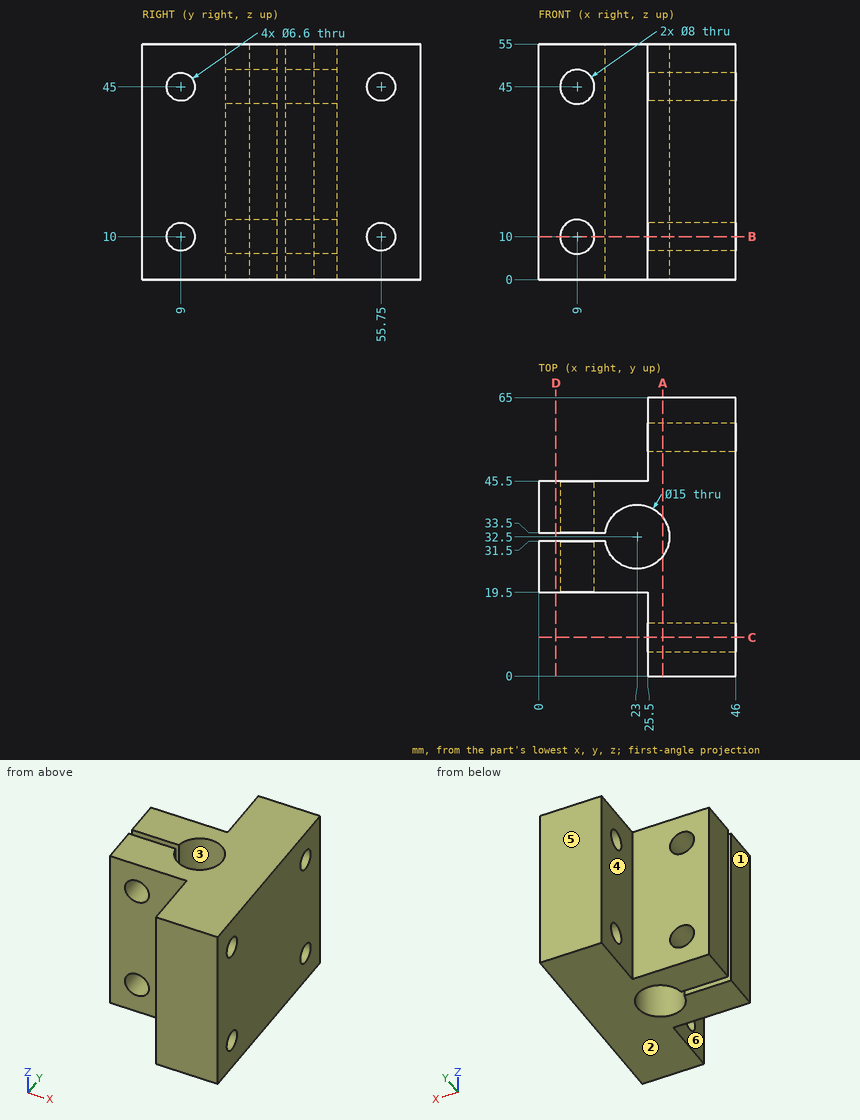
Source: three-view drawing plus pictorial views. Frame: mm from the lowest corner of the part. A direction names the side the tool comes from. Coordinates: 2 decimals unless noted, no trailing zeros. Order: outer loops, then holes, each group sorted by start corner. A loop starts at its lowest first (then second) coordinate and runs counter-clockwise, first axis right, second up. Notation, with made-up numbers: M -24.75,81.25 L -18.75,81.25 A26 ccw -18.75,97.25 Z; hole C 22,19 d3. An arc over 180 degrees is marked long. Write each question's results on one line, items separated by ' | '. Start each with the question number.
1. Pin query (flat end, axial travel): pin 1 (4 mm diameter, centred on y = 55.75, z = 45, fed in from +X); pin 2 (20.5 mm diameter, centred on x = 14.5, z = 37.5, fed in from -Y); pin 3 (10.5 mm diameter, centred on y = 9, z = 10, fed in from -X); pin 4 (13 mm diameter, centred on x = 9, z = 10, fed in from +Y). Return the tip coordinate at first contact, or that it passes through.
2. Section D-D, the plane x = 4. Return the cut outline in (y, z).
3. Section B-B, the plane z = 10. Return the cut outline in (x, y), then the cut area to 3 significant figures.
4. Draft query along X for the marked faces 1, 2 and 3. Return one class per face: +X half, -X half, draft (parallel to the pull), parting line (faces both ways), or undercut.
5. Material intervals for L1, parallel to Z at x = 9, y = 36.5; L2, parallel to Z at x = 37, y = 55; L3, parallel to Y at x = 6.5, z = 51, sorted ascending.
6. Reachability of the marked faces 4, 5 and 6 from +Z, -Z, +X, -X, +Y, -Y: full face, straight path, thin tool, end or side. Return the list, or none.
7. Section A-A, the plane x = 29. Return the cut outline in (y, z), then the cut area to 3 significant figures.
8. Section C-C, the plane y = 9. Return the cut outline in (x, z).
Solution:
1) pin 1: through | pin 2: y = 19.5 | pin 3: x = 25.5 | pin 4: y = 45.5
2) outline: M 19.5,0 L 31.5,0 L 31.5,55 L 19.5,55 Z; M 33.5,0 L 45.5,0 L 45.5,55 L 33.5,55 Z
3) outline: M 0,19.5 L 5,19.5 L 5,31.5 L 0,31.5 Z; M 0,33.5 L 5,33.5 L 5,45.5 L 0,45.5 Z; M 13,19.5 L 25.5,19.5 L 25.5,12.3 L 46,12.3 L 46,52.45 L 25.5,52.45 L 25.5,45.5 L 13,45.5 L 13,33.5 L 15.57,33.5 A7.5 cw long 15.57,31.5 L 13,31.5 Z; M 25.5,0 L 46,0 L 46,5.7 L 25.5,5.7 Z; M 25.5,59.05 L 46,59.05 L 46,65 L 25.5,65 Z | area: 1,330 mm²
4) face 1: -X half | face 2: draft | face 3: undercut
5) L1: 0 to 6, 14 to 41, 49 to 55 | L2: 0 to 6.79, 13.21 to 41.79, 48.21 to 55 | L3: 19.5 to 31.5, 33.5 to 45.5
6) face 4: +Z, -Z, -X, +Y | face 5: +Z, -Z, +X, -X, +Y | face 6: +Z, -Z, -X, -Y
7) outline: M 0,0 L 28,0 L 28,55 L 0,55 Z; M 37,0 L 65,0 L 65,55 L 37,55 Z; hole C 9,10 d6.6; hole C 9,45 d6.6; hole C 55.75,10 d6.6; hole C 55.75,45 d6.6 | area: 2,940 mm²
8) outline: M 25.5,0 L 46,0 L 46,6.7 L 25.5,6.7 Z; M 25.5,13.3 L 46,13.3 L 46,41.7 L 25.5,41.7 Z; M 25.5,48.3 L 46,48.3 L 46,55 L 25.5,55 Z
